Drawing for the job (mm, zero at the part's lowest x, y, z). Round coordinates to 2 decimals unless told otherwise and drop trailing zeros. Loops run counter-clockwise (first coordinate to the right, second up) from the corner with the lowest first, then second, coordinate; pieces in that order, holes last. Notation, with made-up numbers: (-33, -8.75) -> (-3, -8.75) arc R5 cw to (-3, 0.25) -> close; hole circle Ø6 at (57, 82). An arc over 180 degrees is marked (long way). Put each result on its own line as item: value. Start each with the question number.
Item 1: Pull direction Z, two halves, no side cores. Call the marked faces 1 and 2: +Z half, -Z half, draft (parallel to the pull), parting line (faces both ways), or undercut.
Item 2: Cut at A-A, the plane x = 697. List the corners of the cut face in (y, z), plus the area to 3 significant figures.
Item 3: Drill centre lines: probe 1 along X at (y, z) = (31.5, 18.75); probe 2 along Y at (x, z) = (20, 12.25); probe 3 along X at (y, z) = (29, 15). Where is each one in solid material? Low to high. Write a range as [from, to].
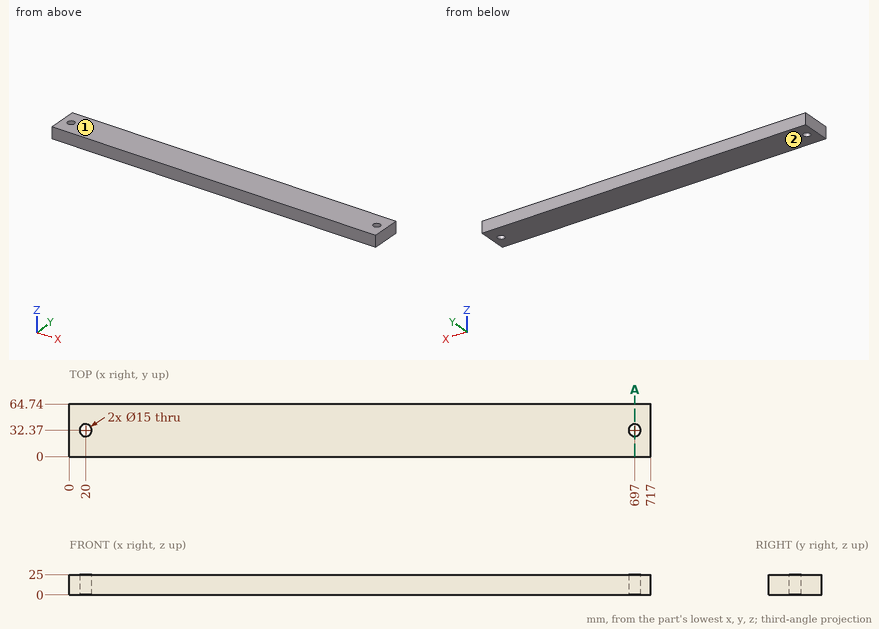
Reply:
1. face 1: +Z half
1. face 2: -Z half
2. outline: (0, 0) -> (24.87, 0) -> (24.87, 25) -> (0, 25) -> close; (39.87, 0) -> (64.74, 0) -> (64.74, 25) -> (39.87, 25) -> close
2. area: 1,240 mm^2
3. probe 1: x = [0, 12.55], [27.45, 689.55], [704.45, 717]
3. probe 2: y = [0, 24.87], [39.87, 64.74]
3. probe 3: x = [0, 13.3], [26.7, 690.3], [703.7, 717]
